Autodesk Inventor part; units mm, degrees
ref_plane "YZ Plane" through (0, 0, 0) normal (1, 0, 0) x (0, 1, 0)
ref_plane "XZ Plane" through (0, 0, 0) normal (0, 1, 0) x (-1, 0, 0)
ref_plane "XY Plane" through (0, 0, 0) normal (0, 0, 1) x (1, 0, 0)
sketch "Sketch1" plane through (0, 0, 0) normal (0, 0, 1) x (1, 0, 0)
  line L0 (-19.05, 0) -> (19.05, 0) construction
  circle A0 centre (-19.05, 0) radius 3.2639
  circle A1 centre (19.05, 0) radius 3.2639
  arc A2 (-25.8481, 6.7981) -> (-28.6639, 0) centre (-19.05, 0) ccw
  arc A3 (28.6639, 0) -> (25.8481, 6.7981) centre (19.05, 0) ccw
  line L1 (-28.6639, 0) -> (-28.6639, -50.8)
  line L2 (-28.6639, -50.8) -> (28.6639, -50.8)
  line L3 (28.6639, -50.8) -> (28.6639, 0)
  line L4 (-25.8481, 6.7981) -> (-2.2451, 30.401)
  line L5 (2.2451, 30.401) -> (25.8481, 6.7981)
  arc A4 (2.2451, 30.401) -> (-2.2451, 30.401) centre (0, 28.156) ccw
  point P0 (0, 0)
  point P1 (0, 0)
  dimension "d0" = 6.5278
  dimension "d1" = 38.1
  dimension "d2" = 6.35
  dimension "d3" = 6.35
  dimension "d4" = 50.8
  dimension "d5" = 3.175
extrude "Extrusion1" add sketch "Sketch1" along normal blind 6.35 contours A0 | A1 | L4 A4 L5 A3 L3 L2 L1 A2
sketch "Sketch2" plane through (0, 0, 6.35) normal (0, 0, 1) x (1, 0, 0)
  line L0 (-19.9009, -41.275) -> (18.1991, -41.275) construction
  line L1 (-28.6639, -50.8) -> (28.6639, -50.8)
  point P0 (0, 0)
  dimension "d8" = 38.1
  dimension "d9" = 9.525
hole "Hole1" at (-19.9009, -41.275, 6.35) at (18.1991, -41.275, 6.35) direction (0, 0, -1) diameter 5.1054 end through all
hole "Hole2" at (-19.05, 0, 0) at (19.05, 0, 0) direction (0, 0, 1) diameter 4.9784 end through all
equation "\"d3\" = d2"
properties part number "CL7-005a" material "Aluminum 6061"
Input: part model. Units: mm. Frame: model coordinates. Give positions to 0.01 mm unless a question says otherwise; leave off trailing zeros. Order: outer loops, then holes, each group sorted by start corner. A loop starts at its lowest first (then second) coordinate and runs counter-clockwise, first axis right, second up. Notation, with made-up numbers: (24, 23) - (56, 23) arc R10 cw to (56, 39) - close; hole circle Ø5 at (44, -4.5). An arc over 180 degrees is marked (long way). Use a Markdown table: item, result.
(1) Line query: line 1 (X direction, y = 0, z = 2.75); line 2 (X direction, y = -39, z = 5.5); line 3 (Y direction, x = 19.05, z = 3.5). Output: solid intervals per line, ascending. Write a range as from..to.
Computed values:
| item | result |
|---|---|
| line 1 | x = -28.66..-21.54, -16.56..16.56, 21.54..28.66 |
| line 2 | x = -28.66..-21.06, -18.74..17.04, 19.36..28.66 |
| line 3 | y = -50.8..-43.68, -38.87..-2.49, 2.49..13.6 |
(2) Section query C-C (y = 11). Output: boundary loops of the cut face in (x, z).
Computed values:
| item | result |
|---|---|
| outline | (-21.65, 0) - (21.65, 0) - (21.65, 6.35) - (-21.65, 6.35) - close |
(3) Section query A-A (x = 19.05). Output: boundary loops of the cut face in (y, z), then the cut area to 3 significant figures.
Computed values:
| item | result |
|---|---|
| outline | (-50.8, 0) - (-43.68, 0) - (-43.68, 6.35) - (-50.8, 6.35) - close; (-38.87, 0) - (-2.49, 0) - (-2.49, 6.35) - (-38.87, 6.35) - close; (2.49, 0) - (13.6, 0) - (13.6, 6.35) - (2.49, 6.35) - close |
| area | 347 mm2 |
(4) Pin query (flat end, axial travel): pin 1 (3 mm diameter, centred on x = -19, y = -41.5, fed in from +Z); pin 2 (1 mm diameter, centred on x = 2.5, z = 5.5, fed in from +Y); pin 3 (2 mm diameter, centred on y = 12, z = 1.5, fed in from +X). Return the tip coordinate at first contact, or that it passes through.
Computed values:
| item | result |
|---|---|
| pin 1 | passes through |
| pin 2 | stops at y = 30.62 |
| pin 3 | stops at x = 21.65 |
(5) Draft query along X for faces 1 (the cylindrical face through (19.752, -39.249, 3.131)), 2 (the cylindrical face through (-0.03, 31.33, 3.13)), 3 (the flat face through (0, -50.8, 3)). Return one class per face: released by +X, released by -X, zero draft, split by the parting line, or undercut.
Computed values:
| item | result |
|---|---|
| face 1 | undercut |
| face 2 | split by the parting line |
| face 3 | zero draft |
(6) Section query B-B (z = 1.75). Output: boundary loops of the cut face in (x, y) (3 decimals).
Computed values:
| item | result |
|---|---|
| outline | (-28.664, -50.8) - (28.664, -50.8) - (28.664, 0) arc R9.614 ccw to (25.848, 6.798) - (2.245, 30.401) arc R3.175 ccw to (-2.245, 30.401) - (-25.848, 6.798) arc R9.614 ccw to (-28.664, 0) - close; hole circle Ø5.105 at (-19.901, -41.275); hole circle Ø4.978 at (-19.05, 0); hole circle Ø5.105 at (18.199, -41.275); hole circle Ø4.978 at (19.05, 0) |
(7) Section query D-D (y = 24). Output: boundary loops of the cut face in (x, z), then the cut area to 3 significant figures.
Computed values:
| item | result |
|---|---|
| outline | (-8.65, 0) - (8.65, 0) - (8.65, 6.35) - (-8.65, 6.35) - close |
| area | 110 mm2 |
